Can you work these out from the drawing? Everything is in mm from the part's minimum corner. Round coordinates to 2 decimals unless told otherwise and drop trailing zeros. Order: outer loops, then holes, each group sorted by start corner. A loop starts at its lowest first (then second) coordinate and runs counter-clockwise, first axis right, second up. Notation, with made-up numbers: (35, -8.75) -> (80, -8.75) arc R21 cw to (80, 19.25) -> close; hole circle Ø1 at (73.5, -27). An arc over 180 degrees is marked (long way). Use a Markdown table: item, result. Add a question column.
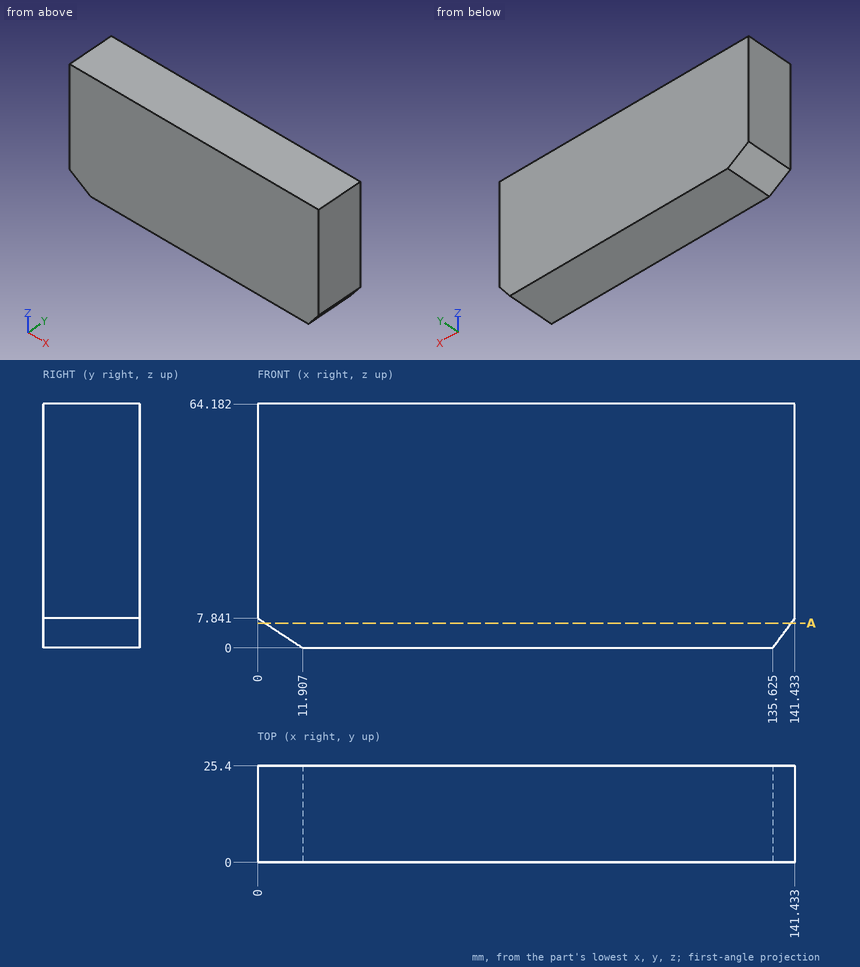
(1) I'm going to push a flat-ended pin straight in: P1, Ø1.5, axis at y = 10.5, z = 19, coming from the -X side. Where does the tip first touch, or does it pass through?
(2) I want a section at A-A on z = 6.5. List the corners of the cut face in (x, y) for me.
(3) Please list where these lines run through material, in increasing order: probe 1 along Z at (x, y) = (136, 19) (1 decimal); probe 2 along Z at (x, y) = (6, 19.25); probe 3 along X at (y, z) = (6.75, 6) (1 decimal). Write a range as from..to.
Output:
| question | item | result |
|---|---|---|
| 1 | P1 | x = 0 |
| 2 | outline | (2.04, 0) -> (140.44, 0) -> (140.44, 25.4) -> (2.04, 25.4) -> close |
| 3 | probe 1 | 0.5..64.2 |
| 3 | probe 2 | 3.89..64.18 |
| 3 | probe 3 | 2.8..140.1 |
